Autodesk Inventor part; units mm, degrees
ref_plane "Work Plane1" through (12.5, 0, 0) normal (1, 0, 0) x (0, 1, 0)
ref_plane "XZ Plane" through (0, 0, 0) normal (0, 1, 0) x (-1, 0, 0)
ref_plane "XY Plane" through (0, 0, 0) normal (0, 0, 1) x (1, 0, 0)
sketch "Sketch1" plane through (0, 0, 0) normal (0, 1, 0) x (-1, 0, 0)
  circle A0 centre (0, 0) radius 7.5
  circle A1 centre (0, 0) radius 2.75
  dimension "d0" = 15
  dimension "d1" = 5.5
extrude "Extrusion1" add sketch "Sketch1" along normal blind 17
sketch "Sketch2" plane through (0, 17, 0) normal (0, 1, 0) x (1, 0, 0)
  circle A0 centre (0, 0) radius 2.75
  circle A1 centre (0, 0) radius 2.75
  circle A2 centre (0, 0) radius 4
  dimension "d4" = 5.5
  dimension "d5" = 8
extrude "Extrusion2" add sketch "Sketch2" along normal blind 7
fillet "Fillet1" radius 6 1 edges at (-4, 17, 0)
fillet "Fillet2" radius 6 2 edges at (0, 17, -7.5) (0, 17, 7.5)
ref_plane "Work Plane1" through (12.5, 0, 0) normal (1, 0, 0) x (0, 1, 0)
mirror "Mirror1" about plane through (12.5, 0, 0) normal (1, 0, 0) of "Extrusion1", "Extrusion2", "Fillet1", "Fillet2"
sketch "Sketch3" plane through (0, 0, 0) normal (0, 1, 0) x (-1, 0, 0)
  circle A0 centre (-25, 0) radius 2.75
  line L0 (-25, 0) -> (-25, 2.75)
  line L1 (-25, 0) -> (-25, -2.75)
  line L2 (0, 0) -> (0, -2.75)
  circle A1 centre (0, 0) radius 2.75
  line L3 (0, 0) -> (0, 2.75)
  line L4 (-25, 2.75) -> (0, 2.75)
  line L5 (0, 2.75) -> (0, 7.5)
  line L6 (0, 7.5) -> (-25, 7.5)
  line L7 (-25, 7.5) -> (-25, 2.75)
  line L8 (-25, -2.75) -> (0, -2.75)
  line L9 (0, -2.75) -> (0, -7.5)
  line L10 (0, -7.5) -> (-25, -7.5)
  line L11 (-25, -7.5) -> (-25, -2.75)
  dimension "d11" = 25
  dimension "d12" = 4.75
  dimension "d13" = 25
  dimension "d14" = 4.75
extrude "Extrusion3" add sketch "Sketch3" along normal blind 11 contours A0 L4 A1 L8 | L7 L6 L5 L4 | L8 L9 L10 L11
sketch "Sketch4" plane through (0, 0, 7.5) normal (0, 0, 1) x (1, 0, 0)
  line L0 (25, 11) -> (0, 11)
  line L1 (12.5, 11) -> (12.5, 6)
  circle A0 centre (12.5, 6) radius 3
  point P0 (0, 0)
  dimension "d17" = 5
  dimension "d18" = 6
extrude "Extrusion4" cut sketch "Sketch4" against normal through all
properties part number "4mm_Roller_Spacer_extended"
Check sheet for the modelled part. Datum: model origin and axes. Units: mm. A direction names the side the tool comes from. Coordinates: 2 decimals unless noted, no trailing zeros. Write each loop counter-clockwise with the first axis right and the second up, starting at its lowest first coordinate (ties: lowest second). Pieces come first, ordered by that corner, then holes. Notation, with made-up numbers: M 73,89.5 L 84,89.5 A14 ccw 84,98.5 Z; hole C -15.5,89.5 d7. An arc over 180 degrees is marked long. Answer as CSV lines item,"result".
Q1. Cross-section at A-A (y = 6). Record the boundary of the cut face in (x, z), then the cut area to 3 significant figures.
Check result:
outline,"M 0,-7.5 L 9.5,-7.5 L 9.5,7.5 L 0,7.5 A7.5 ccw Z; M 15.5,-7.5 L 25,-7.5 A7.5 ccw 25,7.5 L 15.5,7.5 Z; hole C 0,0 d5.5; hole C 25,0 d5.5"
area,"414 mm^2"
Q2. Cross-section at D-D (y = 18.75). Record the boundary of the cut face in (x, z), then the cut area to 3 significant figures.
Check result:
outline,"C 0,0 d10.56; C 25,0 d10.56; hole C 0,0 d5.5; hole C 25,0 d5.5"
area,"128 mm^2"
Q3. Cross-section at C-C (y = 8.5). Record the boundary of the cut face in (x, z), then the cut area to 3 significant figures.
Check result:
outline,"M 0,-7.5 L 10.84,-7.5 L 10.84,7.5 L 0,7.5 A7.5 ccw Z; M 14.16,-7.5 L 25,-7.5 A7.5 ccw 25,7.5 L 14.16,7.5 Z; hole C 0,0 d5.5; hole C 25,0 d5.5"
area,"454 mm^2"
Q4. Cross-section at B-B (x = 12.5). Record the boundary of the cut face in (y, z), then the cut area to 3 significant figures.
Check result:
outline,"M 0,-7.5 L 3,-7.5 L 3,7.5 L 0,7.5 Z; M 9,-7.5 L 11,-7.5 L 11,7.5 L 9,7.5 Z"
area,"75.0 mm^2"
Q5. Material ranges on probe 1 along X at (y, z) = (6, 0); probe 2 along X at (y, z) = (9.25, 0); probe 3 along X at (y, z) = (17, 0), recorded low to high. Write a range as from..to.
Check result:
probe 1,"-7.5..-2.75, 2.75..9.5, 15.5..22.25, 27.75..32.5"
probe 2,"-7.5..-2.75, 2.75..22.25, 27.75..32.5"
probe 3,"-6.69..-2.75, 2.75..6.69, 18.31..22.25, 27.75..31.69"
Q6. Mould release check, pull along Y, two halves, no side actions. Record for faces 3 (the face through (13, 11, 0)), 4 (the face through (10.1, 4.2, 0.1)), 5 (the face through (25.181, 11.832, 2.744)): released by +Y, released by -Y, zero draft, split by the parting line, or undercut.
Check result:
face 3,"released by +Y"
face 4,"undercut"
face 5,"zero draft"
Q7. Set-up check for faces 1 (the face through (-0.867, 23.216, -3.905)), 2 (the face through (3, 24, -1)): record each of +Z, -Z, +X, -X, +Y, -Y from which the full face is reachable in a straight line by a thin tool's end or side.
Check result:
face 1,"+Y"
face 2,"+Z, -Z, +X, -X, +Y"
Q8. Go/stop test with flat-tipped pins: pin 1 (8 mm diameter, centred on x = 0.5, y = 19, fed in from -Z); pin 2 (1 mm diameter, centred on x = 15, z = 4.5, fed in from +Y); pin 3 (5 mm diameter, centred on y = 9.5, z = -3.5, fed in from -X). Record where each tip stops, or that it passes through.
Check result:
pin 1,"z = -7.41"
pin 2,"y = 11"
pin 3,"x = -7.43"
